Here's the drawing with two shaded views (mm, measured from the low corner). I have some questions. A direction names the side the tool comes from. Round coordinates to 2 decimals unless told otherwise and drop trailing zeros. Loops run counter-clockwise (first coordinate to the right, second up) from the corner with the lowest first, then second, coordinate; pieces in that order, holes last. Notation, with made-up numbers: M 88,-33 L 103,-33 A38 cw 103,6 Z; hole C 66,49.5 d3. An arc over 180 degrees is marked long. One line per item, written item: value. Start each with the question number.
Q1. Imagine slicing it at B-B (x = 27). Please give me the cut outline in (y, z) (1 decimal).
Q2. I'm going to push flat-ended pins straight in: pin 1 Ø3 at (x, z) = (51, 14) entering from -Y; pin 2 Ø5 at (x, z) = (76, 7) entering from +Y (1 decimal); pin 3 Ø6 at (x, z) = (72.5, 10.5) entering from +Y. Where does each tip first touch, or does it pass through?
Q3. Thinking about a two-plate mould opening in Y: for the marked faces 3, 4, 5 and 6, which applies, released by +Y, released by -Y, zero draft, split by the parting line, or undercut?
Q4. Please list where these lines run through material, in increasing order: line 1 along X through (y, z) = (101, 8.75) (1 decimal); line 2 along X through (y, z) = (22.5, 8.5) (1 decimal); line 3 along Y through (x, z) = (8.5, 8.25) (1 decimal).
Q5. Imagine slicing it at A-A (y = 102). Please give me the cut outline in (x, z) (1 decimal).
Q6. Imagine slicing it at C-C (z = 17.25). Please give me the cut outline in (x, y) (1 decimal).
Q7. Which directions (+Z, -Z, +X, -X, +Y, -Y) give clear straight access to the entire face, cutting with the end or side of a thin tool? Please do the marked faces 1 and 2.
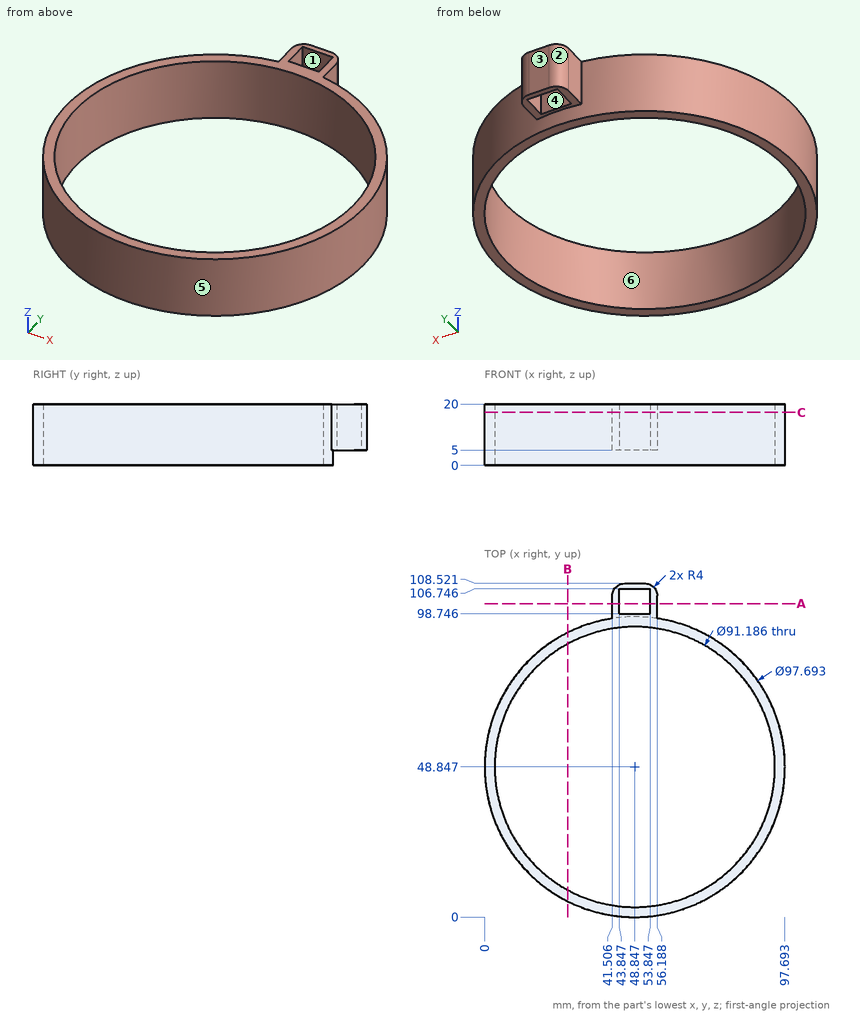
Report:
1. outline: M 5.2,0 L 8.8,0 L 8.8,20 L 5.2,20 Z; M 88.9,0 L 92.5,0 L 92.5,20 L 88.9,20 Z
2. pin 1: stops at y = 0
2. pin 2: stops at y = 91
2. pin 3: stops at y = 93.11
3. face 3: released by +Y
3. face 4: undercut
3. face 5: split by the parting line
3. face 6: undercut
4. line 1: x = 41.5 to 43.8, 53.8 to 56.2
4. line 2: x = 7.7 to 11.6, 86.1 to 90
4. line 3: y = 21.3 to 27.6, 70.1 to 76.4
5. outline: M 41.5,5 L 43.8,5 L 43.8,20 L 41.5,20 Z; M 53.8,5 L 56.2,5 L 56.2,20 L 53.8,20 Z
6. outline: M 41.5,97.1 A48.8 ccw long 56.2,97.1 L 56.2,104.5 A4 ccw 52.2,108.5 L 45.5,108.5 A4 ccw 41.5,104.5 Z; hole C 48.8,48.8 d91.2; hole M 43.8,98.7 L 53.8,98.7 L 53.8,106.7 L 43.8,106.7 Z
7. face 1: +Z, -Z
7. face 2: +Z, -Z, -X, +Y
